```python
from build123d import *

# Parameters (mm, degrees)
CHAMFER1_SIZE = 0.25


with BuildPart() as part:
    # Sketch1 → Revolve1 (revolve)
    with BuildSketch(Plane.XY, mode=Mode.PRIVATE) as revolve1_sk:
        with BuildLine():
            Line((0, 0), (2.5, 0))
            Line((2.5, 0), (2.5, -28))
            Line((2.5, -28), (3.07, -28))
            Line((3.07, -28), (3.07, -29))
            ThreePointArc((3.07, -29), (2.469307539, -31.648711382), (0.784764826, -33.779161865))
            ThreePointArc((0.784764826, -33.779161865), (0.416115665, -33.984911425), (0, -34.05620546))
            Line((0, -34.05620546), (0, 0))
        make_face()
    revolve(revolve1_sk.sketch.rotate(Axis((0, 0, 0), (0, -1, 0)), 180), axis=Axis((0, 0, 0), (0, -1, 0)))

    # Chamfer1
    chamfer1_edges = [part.edges().sort_by_distance(p)[0] for p in [
        (2.5, 0, 0),
    ]]
    chamfer(chamfer1_edges, length=CHAMFER1_SIZE)


solid = part.part
```
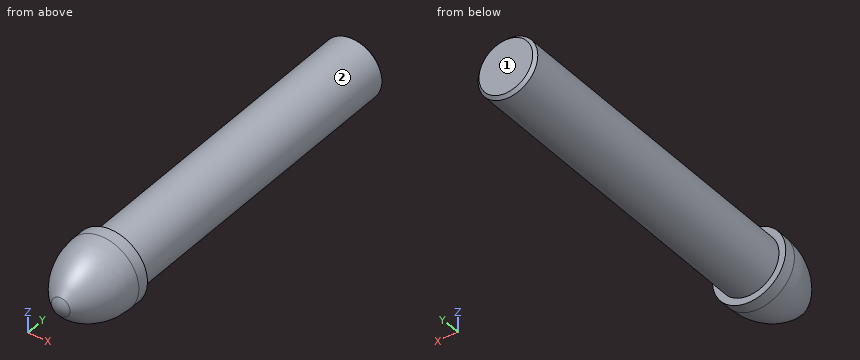
For this review, take the finished solid that the model builds, in its own axes (mm). Face numbers are marked on the shaded views. A direction names the side the tool comes from. Coordinates: 2 decimals unless noted, no trailing zeros. Loops run counter-clockwise (first coordinate to the right, second up) from the corner with the lowest first, then second, coordinate; pieces in that order, holes last.
1. For line 1 (Z direction, x = 0, y = -18.5); line 2 (X direction, y = -5, z = -0.25); line 3 (X direction, y = -26, z = 1), list the stretches that pass through material, from the lowest coordinate up.
2. Add section B-B, the plane y = -5. Give the boundary of the cut face in (x, z), then the cut area to 3 significant figures.
3. For the marked faces 1 and 2, list the 3-axis set-ups (+Z, -Z, +X, -X, +Y, -Y) from which the entire face can be reached by the end or side of a thin tool; tool diameter is ignored.
4. Insertion check: P1, Ø2, axis at x = 0.5, y = -12, coming from the -Z side. The pin has a flat end and moves straight along its axis. Give the tip position at first contact, or say it passes through.
5. Add section A-A, the plane y = -28.5. Give the boundary of the cut face in (x, z).
Result:
1. line 1: z = -2.5 to 2.5
1. line 2: x = -2.49 to 2.49
1. line 3: x = -2.29 to 2.29
2. outline: circle Ø5 at (0, 0)
2. area: 19.6 mm2
3. face 1: +Z, -Z, +X, -X, +Y
3. face 2: +Y
4. P1: stops at z = -2.5
5. outline: circle Ø6.14 at (0, 0)
